Check sheet for the modelled part. Datum: model origin and axes. Units: mm. Give positions to 0.01 mm unless a question says otherwise; leave off trailing zeros. Order: outer loops, then holes, each group sorted by start corner. A loop starts at its lowest first (then second) coordinate and runs counter-clockwise, first axis right, second up. Notation, with made-up numbers: (3, 70) -> (35, 70) arc R19 ccw to (35, 92) -> close; hole circle Ø10 at (-14.5, 36.5). An arc over 180 degrees is marked (long way). Write each question's results on one line, items separated by ' | '.
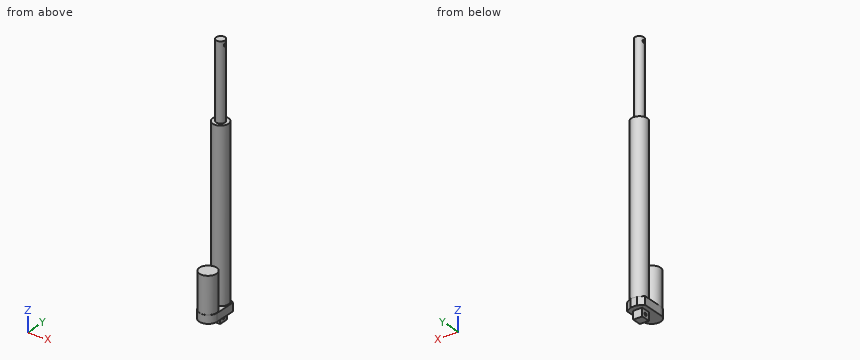
Autodesk Inventor part; units mm, degrees
ref_plane "YZ Plane" through (0, 0, 0) normal (1, 0, 0) x (0, 1, 0)
ref_plane "XZ Plane" through (0, 0, 0) normal (0, 1, 0) x (-1, 0, 0)
ref_plane "XY Plane" through (0, 0, 0) normal (0, 0, 1) x (1, 0, 0)
sketch "Sketch1" plane through (0, 0, 0) normal (0, 0, 1) x (1, 0, 0)
  line L0 (-10, -10) -> (10, -10)
  line L1 (10, -10) -> (10, 10)
  line L2 (10, 10) -> (-10, 10)
  line L3 (-10, 10) -> (-10, -10)
  line L4 (-10, -10) -> (10, 10) construction
  line L5 (10, -10) -> (-10, 10) construction
  line L6 (-20, 15) -> (-20, -32.5)
  line L7 (-20, 15) -> (-7.0096, 22.5)
  line L8 (-20, 15) -> (-5, 15) construction
  line L9 (-7.0096, 22.5) -> (7.0096, 22.5)
  line L10 (7.0096, 22.5) -> (20, 15)
  line L11 (20, 15) -> (20, -32.5)
  circle A0 centre (0, -32.5) radius 20 construction
  arc A1 (-20, -32.5) -> (20, -32.5) centre (0, -32.5) ccw
  point P0 (0, 0)
  point P1 (0, 22.5)
  point P2 (0, 10)
  dimension "d0" = 20
  dimension "d1" = 20
  dimension "d3" = 15
  dimension "d4" = 30
  dimension "d5" = 15
  dimension "d6" = 150
  dimension "d8" = 40
  dimension "d9" = 5
  dimension "d10" = 40
  dimension "d11" = 55
extrude "Extrusion1" add sketch "Sketch1" along normal blind 18
sketch "Sketch2" plane through (0, 0, 18) normal (0, 0, 1) x (1, 0, 0)
  line L0 (-10, -10) -> (-10, 10)
  line L1 (-10, 10) -> (10, 10)
  line L2 (10, 10) -> (10, -10)
  line L3 (10, -10) -> (-10, -10)
  line L4 (-20, 15) -> (-20, -32.5)
  arc A0 (-20, -32.5) -> (20, -32.5) centre (0, -32.5) ccw
  line L5 (20, -32.5) -> (20, 15)
  line L6 (20, 15) -> (7.0096, 22.5)
  line L7 (7.0096, 22.5) -> (-7.0096, 22.5)
  line L8 (-7.0096, 22.5) -> (-20, 15)
  point P0 (0, 0)
extrude "Extrusion2" add sketch "Sketch2" against normal blind 36 contours L0 L1 L2 L3
sketch "Sketch3" plane through (10, -10, 0) normal (1, 0, 0) x (0, 0, -1)
  circle A0 centre (9, 10) radius 3.25
  line L0 (0, 20) -> (18, 20)
  line L1 (0, 0) -> (0, 20)
  point P0 (0, 10)
  point P1 (9, 20)
  point P2 (0, 10)
  dimension "d16" = 6.5
extrude "Extrusion3" cut sketch "Sketch3" against normal through all
sketch "Sketch4" plane through (0, 0, 18) normal (0, 0, 1) x (1, 0, 0)
  circle A0 centre (0, 5) radius 17.5
  line L0 (7.0096, 22.5) -> (-7.0096, 22.5)
  point P0 (0, 0)
  point P1 (0, 22.5)
  dimension "d19" = 35
extrude "Extrusion4" add sketch "Sketch4" along normal blind 369
sketch "Sketch5" plane through (0, 0, 18) normal (0, 0, 1) x (1, 0, 0)
  circle A0 centre (0, -33) radius 19
  circle A1 centre (0, 5) radius 17.5
  point P0 (0, 0)
  dimension "d22" = 38
  dimension "d23" = 38
extrude "Extrusion5" add sketch "Sketch5" along normal blind 80 contours A0
sketch "Sketch10" plane through (0, 5, 387) normal (0, 0, 1) x (1, 0, 0)
  circle A0 centre (0, 0) radius 10
  circle A1 centre (0, 0) radius 17.5
  point P0 (0, -5)
  dimension "d32" = 20
extrude "Extrusion8" add sketch "Sketch10" along normal blind 150 contours A0
sketch "Sketch6" plane through (0, 5, 537) normal (0, 0, 1) x (1, 0, 0)
  circle A0 centre (0, 0) radius 17.5
  circle A1 centre (0, 0) radius 10
  point P0 (0, -5)
  dimension "d26" = 20
extrude "Extrusion6" add sketch "Sketch6" along normal blind 18 contours A1
sketch "Sketch8" plane through (0, 0, 0) normal (1, 0, 0) x (0, 1, 0)
  line L0 (15, 555) -> (-5, 555)
  line L1 (-5, 387) -> (15, 387)
  circle A0 centre (5, 546) radius 3.25
  line L2 (15, 555) -> (-5, 555)
  line L3 (15, 555) -> (15, 537)
  point P0 (0, 0)
  point P1 (5, 387)
  point P2 (15, 546)
  dimension "d29" = 6.5
  dimension "d35" = 18
extrude "Extrusion7" cut sketch "Sketch8" along normal through all both and the other way through all
properties part number "LinearActuator450" material "Steel, Carbon"
1. Section check A-A on z = 29.5. Record the cut outline in (x, y), then the cut area to 3 significant figures.
Verdict:
outline: circle Ø38 at (0, -33); circle Ø35 at (0, 5) | area: 2,100 mm^2
2. Section check C-C on z = 437. Record the cut outline in (x, y).
Verdict:
outline: circle Ø20 at (0, 5)
3. Material ranges on probe 1 along Z at (x, y) = (4, -13); probe 2 along Z at (x, y) = (14.5, 11); probe 3 along Z at (x, y) = (2.25, 5), recorded low to high. Write a range as from..to.
Verdict:
probe 1: z = 0..18 | probe 2: z = 0..387 | probe 3: z = -18..542.75, 549.25..555
4. Section check D-D on z = 329.5. Record the cut outline in (x, y).
Verdict:
outline: circle Ø35 at (0, 5)
5. Gauge pin test, flat ends, axial feed: pin 1 Ø5 at (y, z) = (5, 546) entering from -X; pin 2 Ø6 at (x, y) = (-7.5, 14) entering from -Z; pin 3 Ø10 at (x, z) = (5.5, 387.5) entering from +Y; pin 4 Ø5.5 at (y, z) = (-3, -10.5) entering from +X. Record the tip position at first contact, or that the pin passes through.
Verdict:
pin 1: passes through | pin 2: stops at z = 0 | pin 3: stops at y = 22.49 | pin 4: stops at x = 10
6. Section check B-B on y = -38.5. Record the cut outline in (x, z).
Verdict:
outline: (-19.08, 0) -> (19.08, 0) -> (19.08, 18) -> (18.19, 18) -> (18.19, 98) -> (-18.19, 98) -> (-18.19, 18) -> (-19.08, 18) -> close
